from build123d import *

# Parameters (mm, degrees)
SKETCH2_W          = 11
SKETCH2_H          = 3
CUT_EXTRUDE1_DEPTH = 6


with BuildPart() as part:
    # Sketch1 → Revolve1 (revolve)
    with BuildSketch(Plane.XY):
        Polygon((0, 0), (0, 5), (6.75, 5), (6, 0), align=None)
    revolve(axis=Axis((0, 0, 0), (0, 1, 0)))

    # Sketch2 → Cut-Extrude1 (cut, through all)
    with BuildSketch(Plane(origin=(0, 5, 0), x_dir=(1, 0, 0), z_dir=(0, 1, 0))):
        Rectangle(SKETCH2_W, SKETCH2_H)
    extrude(amount=-CUT_EXTRUDE1_DEPTH, mode=Mode.SUBTRACT)


solid = part.part
Source: CAD feature listing. Evaluate the final solid. Frame: model axes, mm. A direction names the side the tool comes from. Coordinates: 2 decimals unless noted, no trailing zeros. Loops run counter-clockwise (first coordinate to the right, second up) from the corner with the lowest first, then second, coordinate; pieces in that order, holes last. Notation, with made-up numbers: M 36.25,35.5 L 89.25,35.5 A17 cw 89.25,45.5 Z; hole C 41.25,85 d7. An arc over 180 degrees is marked long. Answer in a Markdown table with one row per item.
Q1. Ray query, probe 1 along Z at (x, y) = (1, 1.75); probe 2 along Z at (x, y) = (-5.25, 3.9); probe 3 along X at (y, z) = (2.55, 0.25). Return the intervals inside material, ascending. Write a range as from..to.
Answers below:
| item | result |
|---|---|
| probe 1 | z = -6.18..-1.5, 1.5..6.18 |
| probe 2 | z = -3.97..-1.5, 1.5..3.97 |
| probe 3 | x = -6.38..-5.5, 5.5..6.38 |
Q2. First-contact query: pin 1 (1 mm diameter, centred on x = 5, y = 2.5, fed in from +Z); pin 2 (1.5 mm diameter, centred on x = -3.5, y = 1, fed in from -Z); pin 3 (1.5 mm diameter, centred on x = 2.5, y = 4, fed in from +Z). Flat tips, straight axial feed; report the tip coordinate or a pass-through.
Answers below:
| item | result |
|---|---|
| pin 1 | stops at z = 4.53 |
| pin 2 | stops at z = -5.52 |
| pin 3 | stops at z = 6.39 |
Q3. Section B-B on z = 0. Return the cut outline in (x, y).
Answers below:
| item | result |
|---|---|
| outline | M -6.75,5 L -6,0 L -5.5,0 L -5.5,5 Z; M 5.5,0 L 6,0 L 6.75,5 L 5.5,5 Z |
Q4. Draft query along Z for faces 3 (the conical face through (-1.345, 1.354, 6.056)), 4 (the flat face through (0, 0, 3)), 5 (the flat face through (0, 3, -1.5)). Return one class per face: pulls with the +Z half, pulls with the -Z half, needs draft (parallel to the pull), parting line crosses it, or undercut.
Answers below:
| item | result |
|---|---|
| face 3 | parting line crosses it |
| face 4 | needs draft |
| face 5 | undercut |
Q5. Section D-D on y = 2.35. Return the cut outline in (x, z) (1 decimal), plus the area to 3 significant figures.
Answers below:
| item | result |
|---|---|
| outline | C 0,0 d12.7; hole M -5.5,-1.5 L 5.5,-1.5 L 5.5,1.5 L -5.5,1.5 Z |
| area | 93.8 mm^2 |
Q6. Section A-A on x = 0. Return the cut outline in (y, z), plus the area to 4 significant figures.
Answers below:
| item | result |
|---|---|
| outline | M 0,-6 L 5,-6.75 L 5,-1.5 L 0,-1.5 Z; M 0,1.5 L 5,1.5 L 5,6.75 L 0,6 Z |
| area | 48.75 mm^2 |
Q7. Set-up query: faces 1 (the flat face through (5.5, 3, 0)), 2 (the flat face through (0, 5, -2)). Return all of +Z, -Z, +X, -X, +Y, -Y with unobstructed straight access to the full face (end or side cutting, diameter ignored); none if empty.
Answers below:
| item | result |
|---|---|
| face 1 | +Y, -Y |
| face 2 | +Z, -Z, +X, -X, +Y |
Q8. Section C-C on y = 4.35. Return the cut outline in (x, z) (1 decimal).
Answers below:
| item | result |
|---|---|
| outline | C 0,0 d13.3; hole M -5.5,-1.5 L 5.5,-1.5 L 5.5,1.5 L -5.5,1.5 Z |
